Model file for the job. Use its own axes, mm. A direction names the side the tool comes from. Give positions to 0.01 mm unless a question says otherwise; leave off trailing zeros. Loops run counter-clockwise (first coordinate to the right, second up) from the corner with the lowest first, then second, coordinate; pieces in that order, holes last. Notation, with made-up numbers: (73.25, 18.5) - (92.25, 18.5) arc R17 ccw to (92.25, 33.5) - close; hole circle Ø11 at (28, 6.25). An arc over 180 degrees is marked (long way). Use a Markdown table: item, result.
Autodesk Inventor part; units mm, degrees
ref_plane "YZ Plane" through (0, 0, 0) normal (1, 0, 0) x (0, 1, 0)
ref_plane "XZ Plane" through (0, 0, 0) normal (0, 1, 0) x (-1, 0, 0)
ref_plane "XY Plane" through (0, 0, 0) normal (0, 0, 1) x (1, 0, 0)
ref_plane "Arbeitsebene1" through (0, 0, 0) normal (0, 0, 1) x (1, 0, 0)
sketch "Skizze1" plane through (0, 0, 0) normal (0, 0, 1) x (1, 0, 0)
  line L0 (-2.5, -5) -> (27.5, -5)
  arc A0 (-5, -2.5) -> (-2.5, -5) centre (-2.5, -2.5) ccw
  line L1 (-5, 27.5) -> (-5, -2.5)
  arc A1 (-2.5, 30) -> (-5, 27.5) centre (-2.5, 27.5) ccw
  line L2 (27.5, 30) -> (-2.5, 30)
  arc A2 (30, 27.5) -> (27.5, 30) centre (27.5, 27.5) ccw
  line L3 (30, -2.5) -> (30, 27.5)
  arc A3 (27.5, -5) -> (30, -2.5) centre (27.5, -2.5) ccw
  circle A4 centre (12.5, -9.5) radius 4
  line L4 (30.75, 28.4722) -> (33.3, 29.9445)
  line L5 (33.3, 29.9445) -> (35.85, 28.4722)
  line L6 (35.85, 28.4722) -> (35.85, 25.5278)
  line L7 (35.85, 25.5278) -> (33.3, 24.0555)
  line L8 (33.3, 24.0555) -> (30.75, 25.5278)
  line L9 (30.75, 25.5278) -> (30.75, 28.4722)
  line L10 (25.5278, 30.75) -> (24.0555, 33.3)
  line L11 (24.0555, 33.3) -> (25.5278, 35.85)
  line L12 (25.5278, 35.85) -> (28.4722, 35.85)
  line L13 (28.4722, 35.85) -> (29.9445, 33.3)
  line L14 (29.9445, 33.3) -> (28.4722, 30.75)
  line L15 (28.4722, 30.75) -> (25.5278, 30.75)
  line L16 (30.75, -3.4722) -> (33.3, -4.9445)
  line L17 (30.75, -0.5278) -> (30.75, -3.4722)
  line L18 (33.3, 0.9445) -> (30.75, -0.5278)
  line L19 (35.85, -0.5278) -> (33.3, 0.9445)
  line L20 (35.85, -3.4722) -> (35.85, -0.5278)
  line L21 (33.3, -4.9445) -> (35.85, -3.4722)
  line L22 (25.5278, -5.75) -> (24.0555, -8.3)
  line L23 (28.4722, -5.75) -> (25.5278, -5.75)
  line L24 (29.9445, -8.3) -> (28.4722, -5.75)
  line L25 (28.4722, -10.85) -> (29.9445, -8.3)
  line L26 (25.5278, -10.85) -> (28.4722, -10.85)
  line L27 (24.0555, -8.3) -> (25.5278, -10.85)
  line L28 (-5.75, 28.4722) -> (-8.3, 29.9445)
  line L29 (-5.75, 25.5278) -> (-5.75, 28.4722)
  line L30 (-8.3, 24.0555) -> (-5.75, 25.5278)
  line L31 (-10.85, 25.5278) -> (-8.3, 24.0555)
  line L32 (-10.85, 28.4722) -> (-10.85, 25.5278)
  line L33 (-8.3, 29.9445) -> (-10.85, 28.4722)
  line L34 (-0.5278, 30.75) -> (0.9445, 33.3)
  line L35 (-3.4722, 30.75) -> (-0.5278, 30.75)
  line L36 (-4.9445, 33.3) -> (-3.4722, 30.75)
  line L37 (-3.4722, 35.85) -> (-4.9445, 33.3)
  line L38 (-0.5278, 35.85) -> (-3.4722, 35.85)
  line L39 (0.9445, 33.3) -> (-0.5278, 35.85)
  line L40 (-0.5278, -5.75) -> (0.9445, -8.3)
  line L41 (0.9445, -8.3) -> (-0.5278, -10.85)
  line L42 (-0.5278, -10.85) -> (-3.4722, -10.85)
  line L43 (-3.4722, -10.85) -> (-4.9445, -8.3)
  line L44 (-4.9445, -8.3) -> (-3.4722, -5.75)
  line L45 (-3.4722, -5.75) -> (-0.5278, -5.75)
  line L46 (-5.75, -3.4722) -> (-8.3, -4.9445)
  line L47 (-8.3, -4.9445) -> (-10.85, -3.4722)
  line L48 (-10.85, -3.4722) -> (-10.85, -0.5278)
  line L49 (-10.85, -0.5278) -> (-8.3, 0.9445)
  line L50 (-8.3, 0.9445) -> (-5.75, -0.5278)
  line L51 (-5.75, -0.5278) -> (-5.75, -3.4722)
  circle A5 centre (-9.5, 12.5) radius 4
  line L52 (36.5833, 6.6002) -> (37, 6.6003)
  arc A6 (31.3, 7.45) -> (36.5833, 6.6002) centre (34.01, 7.45) ccw
  line L53 (31.3, 17.55) -> (31.3, 7.45)
  arc A7 (36.5833, 18.3998) -> (31.3, 17.55) centre (34.01, 17.55) ccw
  line L54 (37, 18.3997) -> (36.5833, 18.3998)
  line L55 (37, 35.5) -> (37, 18.3997)
  arc A8 (37, 35.5) -> (35.5, 37) centre (35.5, 35.5) ccw
  line L56 (18.3997, 37) -> (35.5, 37)
  line L57 (18.3998, 36.5833) -> (18.3997, 37)
  arc A9 (17.55, 31.3) -> (18.3998, 36.5833) centre (17.55, 34.01) ccw
  line L58 (7.45, 31.3) -> (17.55, 31.3)
  arc A10 (6.6002, 36.5833) -> (7.45, 31.3) centre (7.45, 34.01) ccw
  line L59 (6.6003, 37) -> (6.6002, 36.5833)
  line L60 (-10.5, 37) -> (6.6003, 37)
  arc A11 (-10.5, 37) -> (-12, 35.5) centre (-10.5, 35.5) ccw
  line L61 (-12, 17) -> (-12, 35.5)
  line L62 (-13.8639, 17) -> (-12, 17)
  arc A12 (-14.6093, 17.6667) -> (-13.8639, 17) centre (-13.8639, 17.75) ccw
  arc A13 (-14.6093, 17.6667) -> (-17.6, 17.5) centre (-16.1, 17.5) ccw
  line L63 (-17.6, 7.5) -> (-17.6, 17.5)
  arc A14 (-17.6, 7.5) -> (-14.6093, 7.3333) centre (-16.1, 7.5) ccw
  arc A15 (-13.8639, 8) -> (-14.6093, 7.3333) centre (-13.8639, 7.25) ccw
  line L64 (-12, 8) -> (-13.8639, 8)
  line L65 (-12, -10.5) -> (-12, 8)
  arc A16 (-12, -10.5) -> (-10.5, -12) centre (-10.5, -10.5) ccw
  line L66 (8, -12) -> (-10.5, -12)
  line L67 (8, -13.8639) -> (8, -12)
  arc A17 (7.3333, -14.6093) -> (8, -13.8639) centre (7.25, -13.8639) ccw
  arc A18 (7.3333, -14.6093) -> (7.5, -17.6) centre (7.5, -16.1) ccw
  line L68 (17.5, -17.6) -> (7.5, -17.6)
  arc A19 (17.5, -17.6) -> (17.6667, -14.6093) centre (17.5, -16.1) ccw
  arc A20 (17, -13.8639) -> (17.6667, -14.6093) centre (17.75, -13.8639) ccw
  line L69 (17, -12) -> (17, -13.8639)
  line L70 (35.5, -12) -> (17, -12)
  arc A21 (35.5, -12) -> (37, -10.5) centre (35.5, -10.5) ccw
  line L71 (37, 6.6003) -> (37, -10.5)
  arc A22 (-18.1, 7.5) -> (-14.1124, 7.2778) centre (-16.1, 7.5) ccw
  arc A23 (-13.8639, 7.5) -> (-14.1124, 7.2778) centre (-13.8639, 7.25) ccw
  line L72 (-18.1, 17.5) -> (-18.1, 7.5)
  line L73 (-12, 8) -> (-13.8639, 8)
  line L74 (-13.8639, 7.5) -> (-13.8639, 8)
  line L75 (-13.8639, 7.5) -> (-12.5, 7.5)
  line L76 (-12, 8) -> (-12.5, 7.5)
  arc A24 (-14.1124, 17.7222) -> (-18.1, 17.5) centre (-16.1, 17.5) ccw
  line L77 (-12.5, 17.5) -> (-13.8639, 17.5)
  arc A25 (-14.1124, 17.7222) -> (-13.8639, 17.5) centre (-13.8639, 17.75) ccw
  line L78 (-12.5, 17.5) -> (-12.5, 7.5)
  point P0 (0, 0)
extrude "Extrusion1" add sketch "Skizze1" along normal blind 5 contours L78 A5 | A5 L78 L64 A15 A14 L63 A13 A12 L62 | L62 A12 A13 L63 A14 A15 L74 A23 A22 L72 A24 A25 L77 L78 | L78 L75 L74 L64 picked at (-12.6815, 11.8821)
mirror "Spiegeln1" about plane through (-12.5, 7.5, 0) normal (1, 0, 0) of "Extrusion1"
chamfer "Fase1" distance 0.5 angle 45 24 edges at (-8.7887, 19.4969, 5) (-6.9, 12.5, 5) (-8.7887, 5.5031, 5) (-10.9694, 7.4363, 5) (-12.5, 7.5, 5) (-14.0306, 7.4363, 5) (-16.2113, 5.5031, 5) (-18.1, 12.5, 5) (-16.2113, 19.4969, 5) (-14.0306, 17.5637, 5) (-12.5, 17.5, 5) (-10.9694, 17.5637, 5) (-12.5, 7.5, 0) (-10.9694, 7.4363, 0) (-8.7887, 5.5031, 0) (-6.9, 12.5, 0) (-8.7887, 19.4969, 0) (-10.9694, 17.5637, 0) (-12.5, 17.5, 0) (-14.0306, 17.5637, 0) (-16.2113, 19.4969, 0) (-18.1, 12.5, 0) (-16.2113, 5.5031, 0) (-14.0306, 7.4363, 0)
properties part number "10_Base_puzzle_nozzle_male_male"
(1) 3-axis set-ups, long thin cutter, end or side, ignore diameter. For faces 4 (the flat face through (-12, 17.5, 2)), 5 (the flat face through (-13, 13, 0)), 6 (the flat face through (-13, 7.5, 2)): which of +Z, -Z, +X, -X, +Y, -Y reach the whole face in a straight line?
Computed:
| item | result |
|---|---|
| face 4 | +Z, -Z, +Y |
| face 5 | -Z, +X, -X, +Y, -Y |
| face 6 | +Z, -Z, -Y |
(2) Slice it at A-A, the plane z = 1. Write the cut outline in (x, y).
Computed:
| item | result |
|---|---|
| outline | (-18.1, 7.5) arc R2 ccw to (-14.11, 7.28) arc R0.25 cw to (-13.86, 7.5) - (-11.14, 7.5) arc R0.25 cw to (-10.89, 7.28) arc R2 ccw to (-6.9, 7.5) - (-6.9, 17.5) arc R2 ccw to (-10.89, 17.72) arc R0.25 cw to (-11.14, 17.5) - (-13.86, 17.5) arc R0.25 cw to (-14.11, 17.72) arc R2 ccw to (-18.1, 17.5) - close |
(3) Slice it at C-C, the plane z = 0.3. Write the cut outline in (x, y), plus the area to 3 significant figures.
Computed:
| item | result |
|---|---|
| outline | (-17.9, 7.5) arc R1.8 ccw to (-14.31, 7.3) arc R0.45 cw to (-13.86, 7.7) - (-11.14, 7.7) arc R0.45 cw to (-10.69, 7.3) arc R1.8 ccw to (-7.1, 7.5) - (-7.1, 17.5) arc R1.8 ccw to (-10.69, 17.7) arc R0.45 cw to (-11.14, 17.3) - (-13.86, 17.3) arc R0.45 cw to (-14.31, 17.7) arc R1.8 ccw to (-17.9, 17.5) - close |
| area | 127 mm² |
(4) Slice it at B-B, the plane x = -12.5. Write the cut outline in (y, z).
Computed:
| item | result |
|---|---|
| outline | (7.5, 0.5) - (8, 0) - (17, 0) - (17.5, 0.5) - (17.5, 4.5) - (17, 5) - (8, 5) - (7.5, 4.5) - close |
(5) Mould opens along X. For faces 1 (the cylindrical face through (-8.83, 19.5, 2.47)), 2 (the flat face through (-13, 13, 5)), 3 (the flat face through (-6.9, 12, 2)) say: pulls with the +X half, pulls with the -X half, needs draft (parallel to the pull), parting line crosses it, or undercut.
Computed:
| item | result |
|---|---|
| face 1 | undercut |
| face 2 | needs draft |
| face 3 | pulls with the +X half |
(6) Pin check, flat tips, straight feed: P1, Ø0.8, axis at x = -12, z = 3, coming from the -Y side; P2, Ø1.4, axis at x = -13, z = 1.5, coming from the +Y side. Stop position of each tip, or through.
Computed:
| item | result |
|---|---|
| P1 | y = 7.5 |
| P2 | y = 17.5 |
(7) Drill centre lines: probe 1 along Y at (x, z) = (-13.5, 0.75); probe 2 along X at (y, z) = (6, 4.65); probe 3 along X at (y, z) = (7, 2.3). Where is each one in solid material? Low to high. Write a range as [from, to].
Computed:
| item | result |
|---|---|
| probe 1 | [7.5, 17.5] |
| probe 2 | [-17.18, -15.02], [-9.98, -7.82] |
| probe 3 | [-18.04, -14.16], [-10.84, -6.96] |
